```python
from build123d import *

# Parameters (mm, degrees)
ESQUISSE1_W             = 170
ESQUISSE1_H             = 40
BOSS_EXTRU_1_DEPTH      = 2
ESQUISSE2_W             = 2
ESQUISSE2_H             = 40
BOSS_EXTRU_2_DEPTH      = 130
ESQUISSE3_W             = 2
ESQUISSE3_H             = 40
BOSS_EXTRU_3_DEPTH      = 130
ESQUISSE4_R             = 2
ENL_V_MAT_EXTRU_1_DEPTH = 171
CONG_1_R                = 1
CONG_2_R                = 1
ESQUISSE5_R             = 3
ENL_V_MAT_EXTRU_2_DEPTH = 130


with BuildPart() as part:
    # Esquisse1 → Boss.-Extru.1 (new body)
    with BuildSketch(Plane.XY):
        with Locations((85, -20)):
            Rectangle(ESQUISSE1_W, ESQUISSE1_H)
    extrude(amount=BOSS_EXTRU_1_DEPTH)

    # Esquisse2 → Boss.-Extru.2 (add)
    with BuildSketch(Plane.XY.offset(2)):
        with Locations((1, -20)):
            Rectangle(ESQUISSE2_W, ESQUISSE2_H)
    extrude(amount=BOSS_EXTRU_2_DEPTH)

    # Esquisse3 → Boss.-Extru.3 (add)
    with BuildSketch(Plane.XY.offset(2)):
        with Locations((169, -20)):
            Rectangle(ESQUISSE3_W, ESQUISSE3_H)
    extrude(amount=BOSS_EXTRU_3_DEPTH)

    # Esquisse4 → Enlèv. mat.-Extru.1 (cut, through all)
    with BuildSketch(Plane.ZY):
        with Locations((112, -20)):
            Circle(ESQUISSE4_R)
    extrude(amount=-ENL_V_MAT_EXTRU_1_DEPTH, mode=Mode.SUBTRACT)

    # Congé1
    cong_1_edges = [part.edges().sort_by_distance(p)[0] for p in [
        (0, -20, 0),
    ]]
    fillet(cong_1_edges, radius=CONG_1_R)

    # Congé2
    cong_2_edges = [part.edges().sort_by_distance(p)[0] for p in [
        (170, -20, 0),
    ]]
    fillet(cong_2_edges, radius=CONG_2_R)

    # Esquisse5 → Enlèv. mat.-Extru.2 (cut)
    with BuildSketch(Plane.XY.offset(2)):
        with Locations((85, -20)):
            Circle(ESQUISSE5_R)
    extrude(amount=-ENL_V_MAT_EXTRU_2_DEPTH, mode=Mode.SUBTRACT)


solid = part.part
```
Check sheet for the modelled part. Datum: model origin and axes. Units: mm. A direction names the side the tool comes from. Round coordinates to 2 decimals unless told otherwise and drop trailing zeros. Order: outer loops, then holes, each group sorted by start corner. A loop starts at its lowest first (then second) coordinate and runs counter-clockwise, first axis right, second up. Notation, with made-up numbers: (5.5, -29) - (33.5, -29) arc R28 cw to (33.5, 3) - close; hole circle Ø5 at (-33.5, 88). An arc over 180 degrees is marked (long way). Answer as CSV lines item,"result". Start each with the question number.
1) Scan lines: probe 1 along X at (y, z) = (-2, 125.5); probe 2 along Y at (x, z) = (169, 112); probe 3 along Z at (x, y) = (150.5, -35.5). Record each from-to range of solid material in increasing order.
2) Section check B-B (x = 85). Record the cut outline in (y, z).
3) Section check D-D (y = -20). Record the cut outline in (x, z).
4) Section check C-C (z = 112). Record the cut outline in (x, y), then the cut area to 3 significant figures.
5) Tool access check on faces 5 (the face through (84, -24, 0)), 6 (the face through (84, -24, 2)). Record the directions out of +Z, -Z, +X, -X, +Y, -Y that give a thin tool (end or side, any length) a straight path to the whole face; none if there is none.
6) Section check A-A (z = 33). Record the cut outline in (x, y).
7) Draft check along X on faces 1 (the face through (170, -20, 66)), 2 (the face through (168, -20, 66)), 3 (the face through (0, -20, 66)), 4 (the face through (1, -20, 110)). Enter one of: +X half, -X half, draft (parallel to the pull), parting line (faces both ways), or undercut.
8) Depth check by flat-ended pin: pin 1 (4 mm diameter, centred on x = 83.5, y = -10.5, fed in from +Z). Enter the tip coordinate at first touch or a pass-through.
Determined:
1,probe 1,"0 to 2, 168 to 170"
1,probe 2,"-40 to -22, -18 to 0"
1,probe 3,"0 to 2"
2,outline,"(-40, 0) - (-23, 0) - (-23, 2) - (-40, 2) - close; (-17, 0) - (0, 0) - (0, 2) - (-17, 2) - close"
3,outline,"(0, 1) arc R1 ccw to (1, 0) - (82, 0) - (82, 2) - (2, 2) - (2, 110) - (0, 110) - close; (0, 114) - (2, 114) - (2, 132) - (0, 132) - close; (88, 0) - (169, 0) arc R1 ccw to (170, 1) - (170, 110) - (168, 110) - (168, 2) - (88, 2) - close; (168, 114) - (170, 114) - (170, 132) - (168, 132) - close"
4,outline,"(0, -40) - (2, -40) - (2, -22) - (0, -22) - close; (0, -18) - (2, -18) - (2, 0) - (0, 0) - close; (168, -40) - (170, -40) - (170, -22) - (168, -22) - close; (168, -18) - (170, -18) - (170, 0) - (168, 0) - close"
4,area,"144 mm^2"
5,face 5,"-Z, +X, -X, +Y, -Y"
5,face 6,"+Z, +Y, -Y"
6,outline,"(0, -40) - (2, -40) - (2, 0) - (0, 0) - close; (168, -40) - (170, -40) - (170, 0) - (168, 0) - close"
7,face 1,"+X half"
7,face 2,"undercut"
7,face 3,"-X half"
7,face 4,"draft"
8,pin 1,"z = 2"
